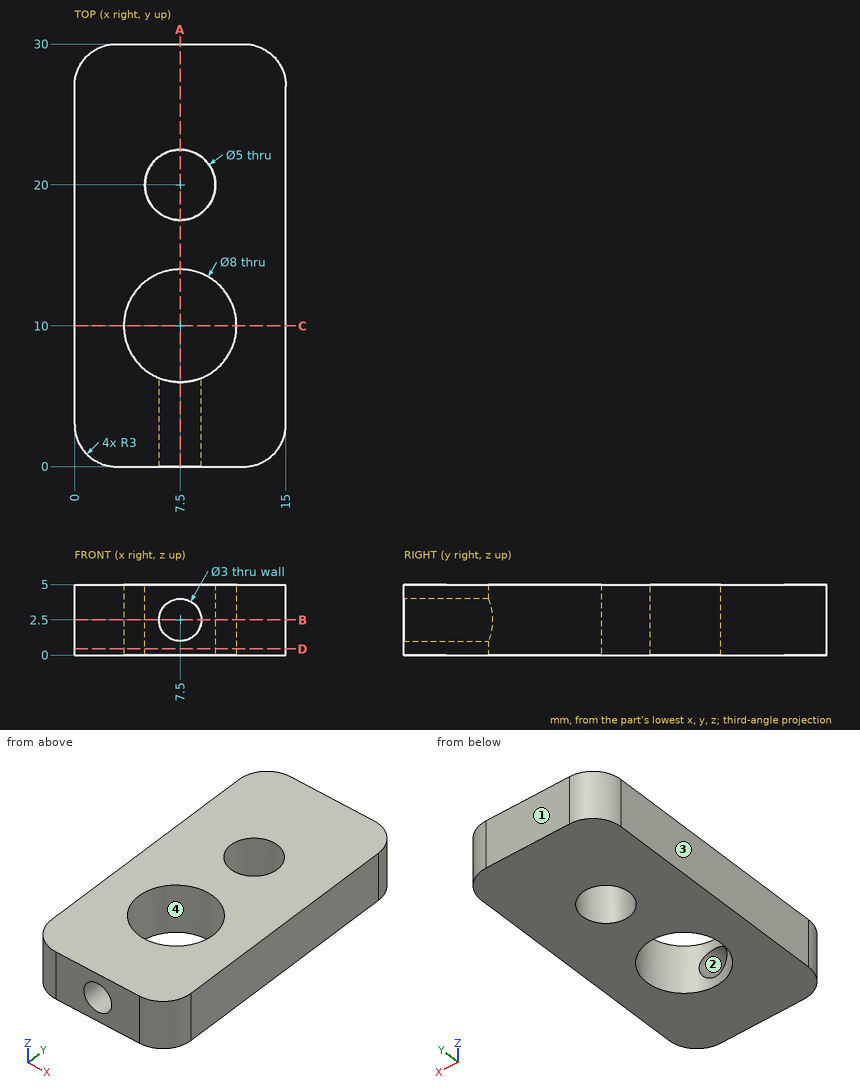
Geometry: see drawing. Coordinates: mm, zero at the bounding-box minimum. Coordinates: 2 decimals unless noted, no trailing zeros. Order: outer loops, then holes, each group sorted by start corner. A loop starts at its lowest first (then second) coordinate and runs counter-clockwise, first axis right, second up. Notation, with made-up numbers: M -27,79 L -5,79 A30 cw -5,113 Z; hole C 24.5,-18 d8. An arc over 180 degrees is marked long. Answer in a Markdown table with one row per item. Add a question column.
Q1. Mould query, pull axis X, two halves, no side actions, for the marked faces 1, 2, 3 and 4. Classes: released by +X, released by -X, zero draft, split by the parting line, or undercut.
Q2. Line query: L1, parallel to Y at x = 7.5, z = 1.3; L2, parallel to Z at x = 7.5, y = 2.5; L3, parallel to X at y = 4, z = 2.5. Output: solid intervals per line, ascending.
Q3. Section query B-B on z = 2.5. Return the cut outline in (x, y).
Q4. Section query C-C on y = 10. Return the cut outline in (x, z).
Q5. Contact query for a flat-ended pin moving along its axis: P1, Ø5, axis at x = 7.5, y = 10, coming from the +Z side. Output: stop coordinate, or through.
Q6. Section query A-A on x = 7.5. Return the cut outline in (y, z).
Q7. Section query D-D on z = 0.45. Return the cut outline in (x, y), and give its area (3 significant figures).
Completed:
| question | item | result |
|---|---|---|
| 1 | face 1 | zero draft |
| 1 | face 2 | undercut |
| 1 | face 3 | released by -X |
| 1 | face 4 | undercut |
| 2 | L1 | y = 14 to 17.5, 22.5 to 30 |
| 2 | L2 | z = 0 to 1, 4 to 5 |
| 2 | L3 | x = 0 to 6, 9 to 15 |
| 3 | outline | M 0,3 A3 ccw 3,0 L 6,0 L 6,6.29 A4 cw long 9,6.29 L 9,0 L 12,0 A3 ccw 15,3 L 15,27 A3 ccw 12,30 L 3,30 A3 ccw 0,27 Z; hole C 7.5,20 d5 |
| 4 | outline | M 0,0 L 3.5,0 L 3.5,5 L 0,5 Z; M 11.5,0 L 15,0 L 15,5 L 11.5,5 Z |
| 5 | P1 | passes through |
| 6 | outline | M 0,0 L 6,0 L 6,1 L 0,1 Z; M 0,4 L 6,4 L 6,5 L 0,5 Z; M 14,0 L 17.5,0 L 17.5,5 L 14,5 Z; M 22.5,0 L 30,0 L 30,5 L 22.5,5 Z |
| 7 | outline | M 0,3 A3 ccw 3,0 L 12,0 A3 ccw 15,3 L 15,27 A3 ccw 12,30 L 3,30 A3 ccw 0,27 Z; hole C 7.5,10 d8; hole C 7.5,20 d5 |
| 7 | area | 372 mm2 |
